Geometry: final body of the model. Coordinates: model frame, mm. A direction names the side the tool comes from. Give positions to 0.01 mm unless a question says otherwise; leave off trailing zeros. Loops run counter-clockwise (first coordinate to the right, second up) from the corner with the lowest first, then second, coordinate; pieces in that order, holes last.
1. Access query for faces 1 (the face through (1, 0, 14)), 2 (the face through (-22.203, 5.067, -0.134)). Directions: +Z, -Z, +X, -X, +Y, -Y. A direction counts if a zero-diameter tool reaches every point of the face in a straight line with its end or side. Return the directions, or none.
2. Section D-D, the plane x = 25. Output: boundary loops of the cut face in (y, z).
3. Draft query along Z for faces 3 (the face through (19.52, 3.94, 62)), 4 (the face through (-15.8, 5, 15.6)), 5 (the face through (1, 8, 28)). Return one class per face: +Z half, -Z half, draft (parallel to the pull), parting line (faces both ways), or undercut.
4. Section C-C, the plane z = 0. Output: boundary loops of the cut face in (x, y), then the cut area to 3 significant figures.
5. Section B-B, the plane x = 0. Output: boundary loops of the cut face in (y, z).
6. Material intervals for line 1 along X through (y, z) = (5.25, -18); line 2 along Z through (x, y) = (-14, 6); line 3 along Y through (x, z) = (-4.5, -20), sorted ascending.
7. First-contact query: P1, Ø4, axis at y = 3.5, z = 25, coming from the +X side; P2, Ø3, axis at y = 4.5, z = 4.5, coming from the +X side; P3, Ø1, axis at y = 3, z = 47.5, coming from the -X side. Flat tips, straight axial feed; report the tip coordinate or a pass-through.
from build123d import *

# Parameters (mm, degrees)
SKETCH1_R           = 65
BOSS_EXTRUDE1_DEPTH = 8
SKETCH2_R           = 10
CUT_EXTRUDE1_DEPTH  = 93.271338995
SKETCH3_R           = 7.026572085
CUT_EXTRUDE2_DEPTH  = 5.949077
CIRPATTERN1_START   = 2.050922526
CIRPATTERN1_DEPTH   = 5.949077474


# Read off the part's stored shape, not the designer's step: CirPattern1
with BuildPart() as part:
    # Sketch1 → Boss-Extrude1 (new body)
    with BuildSketch(Plane(origin=(0, 0, 0), x_dir=(1, 0, 0), z_dir=(0, 1, 0))):
        with Locations(Location((0, 0, 0), (0, 0, 270))):
            Circle(SKETCH1_R)
    extrude(amount=BOSS_EXTRUDE1_DEPTH)

    # Sketch2 → Cut-Extrude1 (cut, through all)
    with BuildSketch(Plane(origin=(0, 0, 0), x_dir=(1, 0, 0), z_dir=(0, 1, 0))):
        with Locations(Location((0, 0, 0), (0, 0, 270))):
            Circle(SKETCH2_R)
    extrude(amount=CUT_EXTRUDE1_DEPTH, mode=Mode.SUBTRACT)

    # Sketch3 → Cut-Extrude2 (cut)
    with BuildSketch(Plane(origin=(0, 8, 0), x_dir=(1, 0, 0), z_dir=(0, 1, 0))):
        with Locations((-15.177293881, 0)):
            Circle(SKETCH3_R)
    extrude(amount=-CUT_EXTRUDE2_DEPTH, mode=Mode.SUBTRACT)

    # CirPattern1 outline → CirPattern1 (cut)
    with BuildSketch(Plane(origin=(0, 0, 0), x_dir=(1, 0, 0), z_dir=(0, 1, 0)).offset(CIRPATTERN1_START)):
        with BuildLine():
            ThreePointArc((3.783785044, -9.256509641), (0, -10), (-3.783785044, -9.256509641))
            ThreePointArc((-3.783785044, -9.256509641), (-3.818273291, -9.278691983), (-3.852631499, -9.301075215))
            ThreePointArc((-3.852631499, -9.301075215), (-3.861099085, -9.260952959), (-3.869800674, -9.220880801))
            ThreePointArc((-3.869800674, -9.220880801), (-7.071067812, -7.071067812), (-9.220880801, -3.869800674))
            ThreePointArc((-9.220880801, -3.869800674), (-9.260952959, -3.861099085), (-9.301075215, -3.852631499))
            ThreePointArc((-9.301075215, -3.852631499), (-12.488341158, -6.491706134), (-16.608186089, -6.879335924))
            ThreePointArc((-16.608186089, -6.879335924), (-15.700504193, -15.700504193), (-6.879335924, -16.608186089))
            ThreePointArc((-6.879335924, -16.608186089), (0, -22.203865966), (6.879335924, -16.608186089))
            ThreePointArc((6.879335924, -16.608186089), (15.700504193, -15.700504193), (16.608186089, -6.879335924))
            ThreePointArc((16.608186089, -6.879335924), (22.203865966, 0), (16.608186089, 6.879335924))
            ThreePointArc((16.608186089, 6.879335924), (15.700504193, 15.700504193), (6.879335924, 16.608186089))
            ThreePointArc((6.879335924, 16.608186089), (0, 22.203865966), (-6.879335924, 16.608186089))
            ThreePointArc((-6.879335924, 16.608186089), (-15.700504193, 15.700504193), (-16.608186089, 6.879335924))
            ThreePointArc((-16.608186089, 6.879335924), (-12.488341158, 6.491706134), (-9.301075215, 3.852631499))
            ThreePointArc((-9.301075215, 3.852631499), (-9.260952959, 3.861099085), (-9.220880801, 3.869800674))
            ThreePointArc((-9.220880801, 3.869800674), (-7.071067812, 7.071067812), (-3.869800674, 9.220880801))
            ThreePointArc((-3.869800674, 9.220880801), (-3.861099085, 9.260952959), (-3.852631499, 9.301075215))
            ThreePointArc((-3.852631499, 9.301075215), (-3.818273291, 9.278691983), (-3.783785044, 9.256509641))
            ThreePointArc((-3.783785044, 9.256509641), (0, 10), (3.783785044, 9.256509641))
            ThreePointArc((3.783785044, 9.256509641), (3.818273291, 9.278691983), (3.852631499, 9.301075215))
            ThreePointArc((3.852631499, 9.301075215), (3.861099085, 9.260952959), (3.869800674, 9.220880801))
            ThreePointArc((3.869800674, 9.220880801), (7.071067812, 7.071067812), (9.220880801, 3.869800674))
            ThreePointArc((9.220880801, 3.869800674), (9.260952959, 3.861099085), (9.301075215, 3.852631499))
            ThreePointArc((9.301075215, 3.852631499), (9.278691983, 3.818273291), (9.256509641, 3.783785044))
            ThreePointArc((9.256509641, 3.783785044), (10, 0), (9.256509641, -3.783785044))
            ThreePointArc((9.256509641, -3.783785044), (9.278691983, -3.818273291), (9.301075215, -3.852631499))
            ThreePointArc((9.301075215, -3.852631499), (9.260952959, -3.861099085), (9.220880801, -3.869800674))
            ThreePointArc((9.220880801, -3.869800674), (7.071067812, -7.071067812), (3.869800674, -9.220880801))
            ThreePointArc((3.869800674, -9.220880801), (3.861099085, -9.260952959), (3.852631499, -9.301075215))
            ThreePointArc((3.852631499, -9.301075215), (3.818273291, -9.278691983), (3.783785044, -9.256509641))
        make_face()
    extrude(amount=CIRPATTERN1_DEPTH, mode=Mode.SUBTRACT)


solid = part.part
Answers below:
1. face 1: +Z, -Z, +X, -X, -Y
1. face 2: +Y
2. outline: (0, -60) - (8, -60) - (8, 60) - (0, 60) - close
3. face 3: parting line
3. face 4: undercut
3. face 5: draft
4. outline: (-65, 0) - (-10, 0) - (-10, 2.05) - (-22.2, 2.05) - (-22.2, 8) - (-65, 8) - close; (10, 0) - (65, 0) - (65, 8) - (22.2, 8) - (22.2, 2.05) - (10, 2.05) - close
4. area: 735 mm2
5. outline: (0, -65) - (8, -65) - (8, -22.2) - (2.05, -22.2) - (2.05, -10) - (0, -10) - close; (0, 10) - (2.05, 10) - (2.05, 22.2) - (8, 22.2) - (8, 65) - (0, 65) - close
6. line 1: x = -62.46 to -6.43, 6.43 to 62.46
6. line 2: z = -63.47 to -16.95, 16.95 to 63.47
6. line 3: y = 0 to 2.05
7. P1: stops at x = 60.79
7. P2: stops at x = 64.93
7. P3: stops at x = -44.9
